from build123d import *

# Parameters (mm, degrees)
F0_W     = 762
F0_H     = 254
F1_DEPTH = 25.4
F3_R     = 12.7
F5_DEPTH = 12.7


# Not quite as in the source:
# - a feature of the source that left no trace in its solid (it failed there, or was rolled back) is left out


with BuildPart() as f1:
    # F0 (on Top) → F1 (new body)
    with BuildSketch(Plane.XY):
        with Locations((-381, -127)):
            Rectangle(F0_W, F0_H)
    extrude(amount=F1_DEPTH)

    # F3
    f3_edges = [f1.edges().sort_by_distance(p)[0] for p in [
        (-762, -254, 12.7),
        (0, -254, 12.7),
        (0, 0, 12.7),
        (0, -127, 25.4),
        (-762, 0, 12.7),
        (-381, 0, 25.4),
        (-762, -127, 25.4),
        (-381, -254, 25.4),
    ]]
    fillet(f3_edges, radius=F3_R)

    # F4 (on face) → F5 (join)
    with BuildSketch(Plane.XY.offset(25.4)):
        with BuildLine():
            Line((-44.45, -165.1), (-38.1, -165.1))
            Line((-38.1, -165.1), (-38.1, -158.75))
            ThreePointArc((-38.1, -158.75), (-42.5901280605, -160.6098719395), (-44.45, -165.1))
        make_face()
        with BuildLine():
            ThreePointArc((-44.45, -165.1), (-38.1, -171.45), (-31.75, -165.1))
            Line((-31.75, -165.1), (-38.1, -165.1))
            Line((-38.1, -165.1), (-44.45, -165.1))
        make_face()
        with BuildLine():
            Line((-38.1, -165.1), (-31.75, -165.1))
            ThreePointArc((-31.75, -165.1), (-33.6098719395, -160.6098719395), (-38.1, -158.75))
            Line((-38.1, -158.75), (-38.1, -165.1))
        make_face()
        with BuildLine():
            Line((-114.3, -165.1), (-107.95, -165.1))
            ThreePointArc((-107.95, -165.1), (-109.8098719395, -160.6098719395), (-114.3, -158.75))
            Line((-114.3, -158.75), (-114.3, -165.1))
        make_face()
        with BuildLine():
            ThreePointArc((-114.3, -158.75), (-118.7901280605, -169.5901280605), (-107.95, -165.1))
            Line((-107.95, -165.1), (-114.3, -165.1))
            Line((-114.3, -165.1), (-114.3, -158.75))
        make_face()
        with BuildLine():
            ThreePointArc((-114.3, -95.25), (-109.8098719395, -93.3901280605), (-107.95, -88.9))
            Line((-107.95, -88.9), (-114.3, -88.9))
            Line((-114.3, -88.9), (-114.3, -95.25))
        make_face()
        with BuildLine():
            Line((-114.3, -88.9), (-107.95, -88.9))
            ThreePointArc((-107.95, -88.9), (-118.7901280605, -84.4098719395), (-114.3, -95.25))
            Line((-114.3, -95.25), (-114.3, -88.9))
        make_face()
        with BuildLine():
            Line((-38.1, -88.9), (-31.75, -88.9))
            ThreePointArc((-31.75, -88.9), (-38.1, -82.55), (-44.45, -88.9))
            Line((-44.45, -88.9), (-38.1, -88.9))
        make_face()
        with BuildLine():
            Line((-38.1, -95.25), (-38.1, -88.9))
            Line((-38.1, -88.9), (-44.45, -88.9))
            ThreePointArc((-44.45, -88.9), (-42.5901280605, -93.3901280605), (-38.1, -95.25))
        make_face()
        with BuildLine():
            ThreePointArc((-38.1, -95.25), (-33.6098719395, -93.3901280605), (-31.75, -88.9))
            Line((-31.75, -88.9), (-38.1, -88.9))
            Line((-38.1, -88.9), (-38.1, -95.25))
        make_face()
    extrude(amount=F5_DEPTH)


solid = f1.part
For this review, take the finished solid that the model builds, in its own axes (mm). Round coordinates to 2 decimals unless told otherwise and drop trailing zeros. Loops run counter-clockwise (first coordinate to the right, second up) from the corner with the lowest first, then second, coordinate; pieces in that order, holes last. Notation, with made-up numbers: (14, -15) - (26, -15) arc R11 cw to (26, -5) - close; hole circle Ø3 at (-25.75, 58.5). An arc over 180 degrees is marked (long way). One line per item, written item: value. Start each with the question number.
Item 1: Clearance check with flat-ended pins moving along their axes: pin 1 Ø12 at (y, z) = (-91, 22) entering from +X; pin 2 Ø1 at (x, y) = (-451.5, -156.5) entering from +Z. State where each tip first meets the part, or that it passes through.
Item 2: Take a section at A-A (x = -154). Give the boundary of the cut face in (y, z).
Item 3: Take a section at B-B (y = -68). Give the boundary of the cut face in (x, z), plus the area to 3 significant figures.
Item 4: For L1, parallel to X at y = -88, z = 36; L2, parallel to Z at x = -66.5, y = -67; L3, parallel to X at y = -57, z = 14, list the stretches that pass through material, from the lowest coordinate up.
Answer below:
1. pin 1: stops at x = -0.44
1. pin 2: stops at z = 25.4
2. outline: (-254, 0) - (0, 0) - (0, 12.7) arc R12.7 ccw to (-12.7, 25.4) - (-241.3, 25.4) arc R12.7 ccw to (-254, 12.7) - close
3. outline: (-762, 0) - (0, 0) - (0, 12.7) arc R12.7 ccw to (-12.7, 25.4) - (-749.3, 25.4) arc R12.7 ccw to (-762, 12.7) - close
3. area: 19,300 mm2
4. L1: x = -120.59 to -108.01, -44.39 to -31.81
4. L2: z = 0 to 25.4
4. L3: x = -761.93 to -0.07
